Verification items for the finished model (mm, model axes). Give positions to 0.01 mm unless a question says otherwise; leave off trailing zeros. Loops run counter-clockwise (first coordinate to the right, second up) from the corner with the lowest first, then second, coordinate; pieces in that order, holes last. Notation, with made-up numbers: M -31.5,29.5 L -19.5,29.5 A5 cw -19.5,33.5 Z; hole C -1,26 d8. An arc over 180 degrees is marked long. Use a Markdown table: item, result.
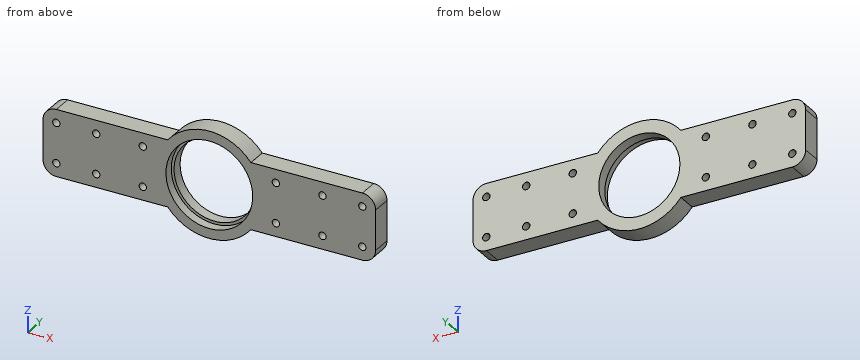
from build123d import *

# Parameters (mm, degrees)
BOSS_EXTRUDE1_DEPTH = 15
CUT_EXTRUDE3_REACH  = 134.098
SKETCH4_R           = 30.5
SKETCH3_R           = 32.6
CUT_EXTRUDE4_DEPTH  = 7
FILLET1_R           = 10


# Read off the part's stored shape, not the designer's step: M5 Clearance Hole1
with BuildPart() as part:
    # Sketch1 → Boss-Extrude1 (new body)
    with BuildSketch(Plane(origin=(0, 0, 0), x_dir=(1, 0, 0), z_dir=(0, 1, 0))):
        with BuildLine():
            ThreePointArc((31.224989992, 25), (0, 40), (-31.224989992, 25))
            Line((-31.224989992, 25), (31.224989992, 25))
        make_face()
        with BuildLine():
            Line((31.224989992, 25), (-31.224989992, 25))
            ThreePointArc((-31.224989992, 25), (-40, 0), (-31.224989992, -25))
            Line((-31.224989992, -25), (31.224989992, -25))
            ThreePointArc((31.224989992, -25), (37.742546282, -13.247648854), (40, 0))
            ThreePointArc((40, 0), (37.742546282, 13.247648854), (31.224989992, 25))
        make_face()
        with BuildLine():
            Line((-31.224989992, 25), (-125, 25))
            Line((-125, 25), (-125, -25))
            Line((-125, -25), (-31.224989992, -25))
            ThreePointArc((-31.224989992, -25), (-40, 0), (-31.224989992, 25))
        make_face()
        with BuildLine():
            Line((125, 25), (31.224989992, 25))
            ThreePointArc((31.224989992, 25), (37.742546282, 13.247648854), (40, 0))
            ThreePointArc((40, 0), (37.742546282, -13.247648854), (31.224989992, -25))
            Line((31.224989992, -25), (125, -25))
            Line((125, -25), (125, 25))
        make_face()
        with BuildLine():
            Line((31.224989992, -25), (-31.224989992, -25))
            ThreePointArc((-31.224989992, -25), (0, -40), (31.224989992, -25))
        make_face()
    extrude(amount=BOSS_EXTRUDE1_DEPTH)

    # Sketch4 → Cut-Extrude3 (cut, up to next)
    with BuildSketch(Plane(origin=(0, 15, 0), x_dir=(1, 0, 0), z_dir=(0, 1, 0)), mode=Mode.PRIVATE) as cut_extrude3_sk1:
        with Locations(Location((0, 0, 0), (0, 0, 270))):
            Circle(SKETCH4_R)
    cut_extrude3_tool1 = extrude(cut_extrude3_sk1.sketch, amount=-CUT_EXTRUDE3_REACH, mode=Mode.PRIVATE) & part.part
    add(cut_extrude3_tool1.solids().sort_by_distance((0, 15, 0))[0], mode=Mode.SUBTRACT)

    # Sketch3 → Cut-Extrude4 (cut)
    with BuildSketch(Plane.XZ):
        with Locations(Location((0, 0, 0), (0, 0, 270))):
            Circle(SKETCH3_R)
    extrude(amount=-CUT_EXTRUDE4_DEPTH, mode=Mode.SUBTRACT)

    # M5 Clearance Hole1 outline → M5 Clearance Hole1 (revolve, cut)
    with BuildSketch(Plane(origin=(-50, 0, 15), x_dir=(1, 0, 0), z_dir=(0, 0, 1))):
        Polygon((0, 0), (2.75, 0), (2.75, 14.975), (2.775, 15), (0, 15), align=None)
    revolve(axis=Axis((-50, 0, 15), (0, 1, 0)), mode=Mode.SUBTRACT)

    # M5 Clearance Hole1 2 outline → M5 Clearance Hole1 2 (revolve, cut)
    with BuildSketch(Plane(origin=(-50, 0, -15), x_dir=(1, 0, 0), z_dir=(0, 0, 1))):
        Polygon((0, 0), (2.75, 0), (2.75, 14.975), (2.775, 15), (0, 15), align=None)
    revolve(axis=Axis((-50, 0, -15), (0, 1, 0)), mode=Mode.SUBTRACT)

    # M5 Clearance Hole1 3 outline → M5 Clearance Hole1 3 (revolve, cut)
    with BuildSketch(Plane(origin=(50, 0, 15), x_dir=(1, 0, 0), z_dir=(0, 0, 1))):
        Polygon((0, 0), (2.75, 0), (2.75, 14.975), (2.775, 15), (0, 15), align=None)
    revolve(axis=Axis((50, 0, 15), (0, 1, 0)), mode=Mode.SUBTRACT)

    # M5 Clearance Hole1 4 outline → M5 Clearance Hole1 4 (revolve, cut)
    with BuildSketch(Plane(origin=(50, 0, -15), x_dir=(1, 0, 0), z_dir=(0, 0, 1))):
        Polygon((0, 0), (2.75, 0), (2.75, 14.975), (2.775, 15), (0, 15), align=None)
    revolve(axis=Axis((50, 0, -15), (0, 1, 0)), mode=Mode.SUBTRACT)

    # M5 Clearance Hole1 5 outline → M5 Clearance Hole1 5 (revolve, cut)
    with BuildSketch(Plane(origin=(115, 0, -15), x_dir=(1, 0, 0), z_dir=(0, 0, 1))):
        Polygon((0, 0), (2.75, 0), (2.75, 14.975), (2.775, 15), (0, 15), align=None)
    revolve(axis=Axis((115, 0, -15), (0, 1, 0)), mode=Mode.SUBTRACT)

    # M5 Clearance Hole1 6 outline → M5 Clearance Hole1 6 (revolve, cut)
    with BuildSketch(Plane(origin=(85, 0, 15), x_dir=(1, 0, 0), z_dir=(0, 0, 1))):
        Polygon((0, 0), (2.75, 0), (2.75, 14.975), (2.775, 15), (0, 15), align=None)
    revolve(axis=Axis((85, 0, 15), (0, 1, 0)), mode=Mode.SUBTRACT)

    # M5 Clearance Hole1 7 outline → M5 Clearance Hole1 7 (revolve, cut)
    with BuildSketch(Plane(origin=(115, 0, 15), x_dir=(1, 0, 0), z_dir=(0, 0, 1))):
        Polygon((0, 0), (2.75, 0), (2.75, 14.975), (2.775, 15), (0, 15), align=None)
    revolve(axis=Axis((115, 0, 15), (0, 1, 0)), mode=Mode.SUBTRACT)

    # M5 Clearance Hole1 8 outline → M5 Clearance Hole1 8 (revolve, cut)
    with BuildSketch(Plane(origin=(85, 0, -15), x_dir=(1, 0, 0), z_dir=(0, 0, 1))):
        Polygon((0, 0), (2.75, 0), (2.75, 14.975), (2.775, 15), (0, 15), align=None)
    revolve(axis=Axis((85, 0, -15), (0, 1, 0)), mode=Mode.SUBTRACT)

    # M5 Clearance Hole1 9 outline → M5 Clearance Hole1 9 (revolve, cut)
    with BuildSketch(Plane(origin=(-85, 0, -15), x_dir=(1, 0, 0), z_dir=(0, 0, 1))):
        Polygon((0, 0), (2.75, 0), (2.75, 14.975), (2.775, 15), (0, 15), align=None)
    revolve(axis=Axis((-85, 0, -15), (0, 1, 0)), mode=Mode.SUBTRACT)

    # M5 Clearance Hole1 10 outline → M5 Clearance Hole1 10 (revolve, cut)
    with BuildSketch(Plane(origin=(-115, 0, 15), x_dir=(1, 0, 0), z_dir=(0, 0, 1))):
        Polygon((0, 0), (2.75, 0), (2.75, 14.975), (2.775, 15), (0, 15), align=None)
    revolve(axis=Axis((-115, 0, 15), (0, 1, 0)), mode=Mode.SUBTRACT)

    # M5 Clearance Hole1 11 outline → M5 Clearance Hole1 11 (revolve, cut)
    with BuildSketch(Plane(origin=(-85, 0, 15), x_dir=(1, 0, 0), z_dir=(0, 0, 1))):
        Polygon((0, 0), (2.75, 0), (2.75, 14.975), (2.775, 15), (0, 15), align=None)
    revolve(axis=Axis((-85, 0, 15), (0, 1, 0)), mode=Mode.SUBTRACT)

    # M5 Clearance Hole1 12 outline → M5 Clearance Hole1 12 (revolve, cut)
    with BuildSketch(Plane(origin=(-115, 0, -15), x_dir=(1, 0, 0), z_dir=(0, 0, 1))):
        Polygon((0, 0), (2.75, 0), (2.75, 14.975), (2.775, 15), (0, 15), align=None)
    revolve(axis=Axis((-115, 0, -15), (0, 1, 0)), mode=Mode.SUBTRACT)

    # Fillet1
    fillet1_edges = [part.edges().sort_by_distance(p)[0] for p in [
        (125, 7.5, -25),
        (125, 7.5, 25),
        (-125, 7.5, 25),
        (-125, 7.5, -25),
    ]]
    fillet(fillet1_edges, radius=FILLET1_R)


solid = part.part
(1) Cross-section at A-A on z = 0. Record the cut outline in (x, y).
Results below:
| item | result |
|---|---|
| outline | M -125,0 L -32.6,0 L -32.6,7 L -30.5,7 L -30.5,15 L -125,15 Z; M 30.5,7 L 32.6,7 L 32.6,0 L 125,0 L 125,15 L 30.5,15 Z |
(2) Cross-section at B-B on y = 4. State how many separate pieces and enclosed holes the cut face has, then the cut area to 3 significant figures.
Results below:
| item | result |
|---|---|
| separate pieces | 1 |
| enclosed holes | 13 |
| area | 10,100 mm^2 |
(3) Material ranges on line 1 (Z direction, x = -115, y = 11.5); line 2 (X direction, y = 9.25, z = 0); line 3 (Z direction, x = 52, y = 11.5), recorded low to high.
Results below:
| item | result |
|---|---|
| line 1 | -25 to -17.75, -12.25 to 12.25, 17.75 to 25 |
| line 2 | -125 to -30.5, 30.5 to 125 |
| line 3 | -25 to -16.89, -13.11 to 13.11, 16.89 to 25 |
(4) Cross-section at C-C on x = 85. Record the cut outline in (y, z) (3 decimals), then the cut area to 3 significant figures.
Results below:
| item | result |
|---|---|
| outline | M 0,-25 L 15,-25 L 15,-17.775 L 14.975,-17.75 L 0,-17.75 Z; M 0,-12.25 L 14.975,-12.25 L 15,-12.225 L 15,12.225 L 14.975,12.25 L 0,12.25 Z; M 0,17.75 L 14.975,17.75 L 15,17.775 L 15,25 L 0,25 Z |
| area | 585 mm^2 |
(5) Cross-section at D-D on x = 0. Record the cut outline in (y, z), then the cut area to 3 significant figures.
Results below:
| item | result |
|---|---|
| outline | M 0,-40 L 15,-40 L 15,-30.5 L 7,-30.5 L 7,-32.6 L 0,-32.6 Z; M 0,32.6 L 7,32.6 L 7,30.5 L 15,30.5 L 15,40 L 0,40 Z |
| area | 256 mm^2 |
(6) Gauge pin test, flat ends, axial feed: P1, Ø1.5, axis at x = 73, y = 2.5, coming from the -Z side; P2, Ø4.5, axis at x = -115, z = -15, coming from the +Y side; P3, Ø4.5, axis at x = 67.5, y = 4, coming from the +Z side; P4, Ø4, axis at y = 4.5, z = -29.5, coming from the +X side. Record the tip position at first contact, or that the pin passes through.
Results below:
| item | result |
|---|---|
| P1 | z = -25 |
| P2 | through |
| P3 | z = 25 |
| P4 | x = 29.05 |
